```python
from build123d import *

# Parameters (mm, degrees)
SKETCH1_R           = 3.5
BOSS_EXTRUDE1_DEPTH = 1
SKETCH2_R           = 5.5
BOSS_EXTRUDE2_DEPTH = 8
SKETCH3_R           = 5.5
BOSS_EXTRUDE3_DEPTH = 9
BOSS_EXTRUDE5_DEPTH = 10
SKETCH5_R           = 1.5
CUT_EXTRUDE1_DEPTH  = 30.060282173
SKETCH6_R           = 2.6
CUT_EXTRUDE2_DEPTH  = 3.1
SKETCH7_R           = 8.67620316
SKETCH7_R_2         = 3.225
CUT_EXTRUDE3_DEPTH  = 3
CUT_EXTRUDE4_START  = -3.1
SKETCH8_R           = 2.6
CUT_EXTRUDE4_DEPTH  = 3.1


with BuildPart() as part:
    # Sketch1 → Boss-Extrude1 (new body)
    with BuildSketch(Plane(origin=(0, 0, 0), x_dir=(1, 0, 0), z_dir=(0, 1, 0))):
        with Locations(Location((0, 0, 0), (0, 0, 270))):
            Circle(SKETCH1_R)
    extrude(amount=BOSS_EXTRUDE1_DEPTH)

    # Sketch2 → Boss-Extrude2 (add)
    with BuildSketch(Plane(origin=(0, 1, 0), x_dir=(1, 0, 0), z_dir=(0, 1, 0))):
        with Locations(Location((0, 0, 0), (0, 0, 270))):
            Circle(SKETCH2_R)
    extrude(amount=BOSS_EXTRUDE2_DEPTH)

    # Sketch3 → Boss-Extrude3 (add)
    with BuildSketch(Plane(origin=(0, 9, 0), x_dir=(1, 0, 0), z_dir=(0, 1, 0))):
        with Locations(Location((0, 0, 0), (0, 0, 270))):
            Circle(SKETCH3_R)
    extrude(amount=BOSS_EXTRUDE3_DEPTH)

    # Sketch4 → Boss-Extrude5 (add)
    with BuildSketch(Plane(origin=(0, 18, 0), x_dir=(1, 0, 0), z_dir=(0, 1, 0))):
        Polygon((3.277230323, -1.768406461), (3.170100081, 1.953961483), (-0.107130242, 3.722367944), (-3.277230323, 1.768406461), (-3.170100081, -1.953961483), (0.107130242, -3.722367944), align=None)
    extrude(amount=BOSS_EXTRUDE5_DEPTH)

    # Sketch5 → Cut-Extrude1 (cut, through all)
    with BuildSketch(Plane(origin=(0, 28, 0), x_dir=(1, 0, 0), z_dir=(0, 1, 0))):
        with Locations(Location((0, 0, 0), (0, 0, 270))):
            Circle(SKETCH5_R)
    extrude(amount=-CUT_EXTRUDE1_DEPTH, mode=Mode.SUBTRACT)

    # Sketch6 → Cut-Extrude2 (cut)
    with BuildSketch(Plane.XZ):
        with Locations(Location((0, 0, 0), (0, 0, 270))):
            Circle(SKETCH6_R)
    extrude(amount=-CUT_EXTRUDE2_DEPTH, mode=Mode.SUBTRACT)

    # Sketch7 → Cut-Extrude3 (cut)
    with BuildSketch(Plane(origin=(0, 10.1, 0), x_dir=(1, 0, 0), z_dir=(0, 1, 0))):
        Circle(SKETCH7_R)
        with Locations(Location((0, 0, 0), (0, 0, 270))):
            Circle(SKETCH7_R_2, mode=Mode.SUBTRACT)
    extrude(amount=CUT_EXTRUDE3_DEPTH, mode=Mode.SUBTRACT)

    # Sketch8 → Cut-Extrude4 (cut)
    with BuildSketch(Plane(origin=(0, 28, 0), x_dir=(1, 0, 0), z_dir=(0, 1, 0)).offset(CUT_EXTRUDE4_START)):
        with Locations(Location((0, 0, 0), (0, 0, 90))):
            Circle(SKETCH8_R)
    extrude(amount=CUT_EXTRUDE4_DEPTH, mode=Mode.SUBTRACT)


solid = part.part
```
Source: CAD feature listing. Evaluate the final solid. Frame: model axes, mm. A direction names the side the tool comes from. Give positions to 0.01 mm unless a question says otherwise; leave off trailing zeros. Write each loop counter-clockwise with the first axis right and the second up, starting at its lowest first coordinate (ties: lowest second). Pieces come first, ordered by that corner, then holes.
1. Section query A-A (y = 18.5). Return the cut outline in (x, z).
2. Pull-direction query (Z, two-part tool) for faces 1 (the face through (2.4, 13.1, 2.4)), 2 (the face through (0, 24.9, -2)), 3 (the face through (-1.67, 22.93, -2.76)); classes: +Z half, -Z half, draft (parallel to the pull), parting line (faces both ways), or undercut.
3. First-contact query: pin 1 (2 mm diameter, centred on x = 3.5, y = 24.5, fed in from -Z); pin 2 (3.5 mm diameter, centred on x = 1, z = -2.5, fed in from -Y); pin 3 (2 mm diameter, centred on y = 4, z = 3.5, fed in from -X); pin 4 (5 mm diameter, centred on x = 0, z = 0, fed in from -Y). Flat tips, straight axial feed; report the tip coordinate or a pass-through.
4. Section query C-C (x = 4.25). Return the cut outline in (y, z), then the cut area to 3 significant figures.
5. Material intervals for line 1 along X through (y, z) = (27, 0); line 2 along X through (y, z) = (0.95, 0); line 3 along Y through (x, z) = (-2.5, 4.75), sorted ascending.
6. Access query for faces 4 (the face through (-3.417, 0.493, -0.759)), 5 (the face through (-3.15, 11.58, -0.7)), 6 (the face through (-1.6, 22.9, 2.8)), 7 (the face through (-2, 18, -3)), 8 (the face through (1.6, 22.9, -2.8)). Directions: +Z, -Z, +X, -X, +Y, -Y. A direction counts if a zero-diameter tool reaches every point of the face in a straight line with its end or side. Return the directions, or none.
7. Section query D-D (y = 25.5). Return the cut outline in (x, z).
Output values:
1. outline: (-3.28, -1.77) - (-0.11, -3.72) - (3.17, -1.95) - (3.28, 1.77) - (0.11, 3.72) - (-3.17, 1.95) - close; hole circle Ø3 at (0, 0)
2. face 1: draft
2. face 2: undercut
2. face 3: -Z half
3. pin 1: stops at z = -2.32
3. pin 2: stops at y = 0
3. pin 3: stops at x = -4.9
3. pin 4: stops at y = 3.1
4. outline: (1, -3.49) - (10.1, -3.49) - (10.1, 3.49) - (1, 3.49) - close; (13.1, -3.49) - (18, -3.49) - (18, 3.49) - (13.1, 3.49) - close
4. area: 97.7 mm2
5. line 1: x = -3.23 to -2.6, 2.6 to 3.23
5. line 2: x = -3.5 to -2.6, 2.6 to 3.5
5. line 3: y = 1 to 10.1, 13.1 to 18
6. face 4: -Y
6. face 5: none
6. face 6: +Z, -X, +Y
6. face 7: +Y
6. face 8: -Z, +X, +Y
7. outline: (-3.28, -1.77) - (-0.11, -3.72) - (3.17, -1.95) - (3.28, 1.77) - (0.11, 3.72) - (-3.17, 1.95) - close; hole circle Ø5.2 at (0, 0)
